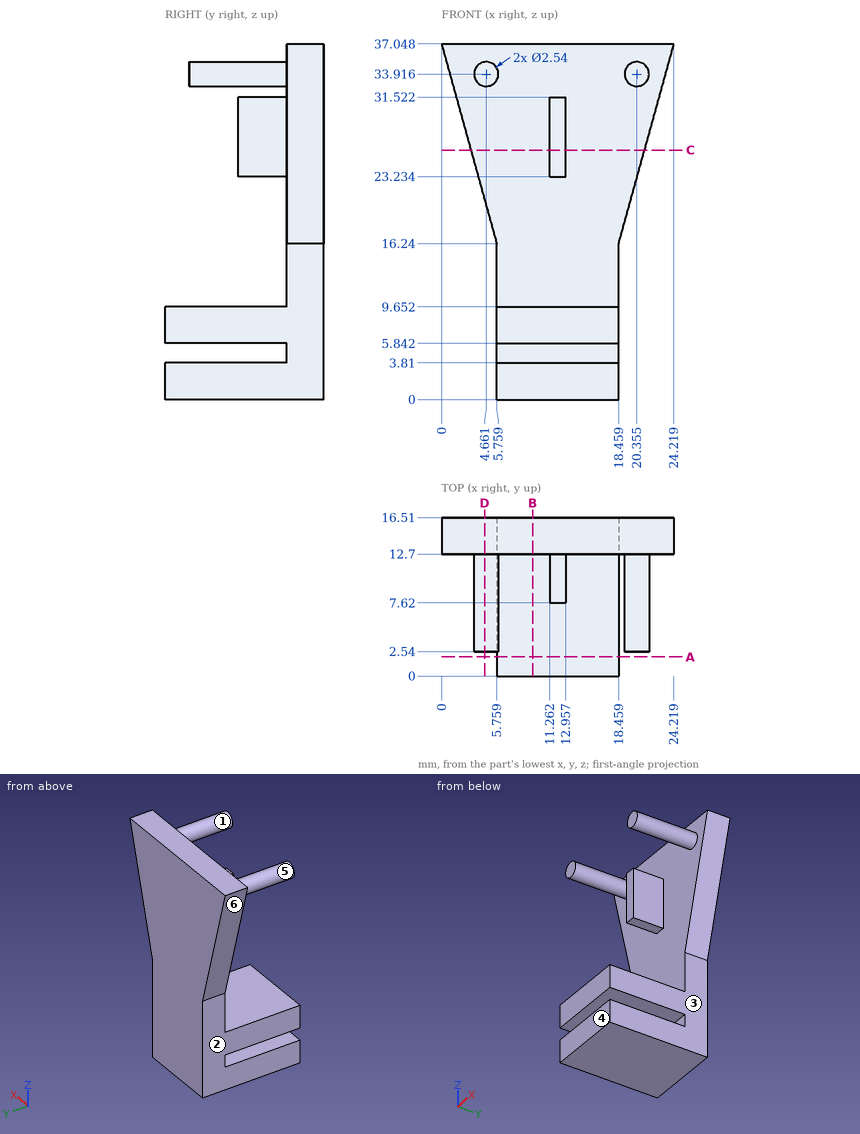
For this review, use the dimensioned drawing (mm, ordinates from the lowest corner) and the shaded views. A direction names the side the tool comes from. Give positions to 0.01 mm unless a question says otherwise; leave off trailing zeros. Order: outer loops, then holes, each group sorted by start corner. A loop starts at its lowest first (then second) coordinate and runs counter-clockwise, first axis right, second up. Notation, with made-up numbers: M -21,-15 L -17,-15 A16 ccw -17,6 Z; hole C -14,58 d3. An arc over 180 degrees is marked long. One line per question, with ' | ' between items. Start each with the question number.
1) Consider section D-D, the plane x = 4.5. Give the boundary of the cut face in (y, z) (1 decimal).
2) Clearance check with flat-ended pins moving along their axes: P1, Ø3, axis at x = 20, z = 33.5, coming from the -Y side; P2, Ø1.4, axis at x = 12, y = 10.5, coming from the +Z side; P3, Ø12, axis at x = 12, z = 26.5, coming from the -Y side; P4, Ø1.9, axis at x = 12, y = 10.5, coming from the -Z side. State where each tip first meets the part, or that it passes through.
3) Wall thickness on L1, parallel to Z at x = 10.5, y = 4.5; L2, parallel to X at y = 14.25, z = 8.5; L3, parallel to Y at x = 16.75, z = 35.5: over which ranges is each line inside the solid? List them lowest first. Write a range as from..to.
4) For the marked faces 1, 2 and 3, list the 3-axis set-ups (+Z, -Z, +X, -X, +Y, -Y) from which the entire face can be reached by the end or side of a thin tool; tool diameter is ignored.
5) Consider section A-A, the plane y = 2. Give the boundary of the cut face in (x, z).
6) Consider section C-C, the plane z = 26. Give the boundary of the cut face in (x, y).
7) Consider section B-B, the plane x = 9.5. Give the boundary of the cut face in (y, z), then the cut area to 3 significant figures.
8) Mouldability with a two-part tool opening along X and no side actions: class the marked faces 4, 5 and 6 as pulls with the +X half, pulls with the -X half, needs draft (parallel to the pull), parting line crosses it, or undercut.
Found:
1) outline: M 2.5,32.7 L 12.7,32.7 L 12.7,20.8 L 16.5,20.8 L 16.5,37 L 12.7,37 L 12.7,35.2 L 2.5,35.2 Z
2) P1: stops at y = 2.54 | P2: stops at z = 31.52 | P3: stops at y = 7.62 | P4: stops at z = 0
3) L1: z = 0..3.81, 5.84..9.65 | L2: x = 5.76..18.46 | L3: y = 12.7..16.51
4) face 1: -Y | face 2: -Z, -X, +Y, -Y | face 3: -Z, +X, +Y, -Y
5) outline: M 5.76,0 L 18.46,0 L 18.46,3.81 L 5.76,3.81 Z; M 5.76,5.84 L 18.46,5.84 L 18.46,9.65 L 5.76,9.65 Z
6) outline: M 3.06,12.7 L 11.26,12.7 L 11.26,7.62 L 12.96,7.62 L 12.96,12.7 L 21.16,12.7 L 21.16,16.51 L 3.06,16.51 Z
7) outline: M 0,0 L 16.51,0 L 16.51,37.05 L 12.7,37.05 L 12.7,9.65 L 0,9.65 L 0,5.84 L 12.7,5.84 L 12.7,3.81 L 0,3.81 Z | area: 238 mm²
8) face 4: needs draft | face 5: undercut | face 6: pulls with the -X half
